Part print with two shaded views. Sizes in mm from the minimum x, y, z corner. A direction names the side the tool comes from. Coordinates: 2 decimals unless noted, no trailing zeros. Loops run counter-clockwise (first coordinate to the right, second up) from the corner with the lowest first, then second, coordinate; pieces in that order, holes last. Notation, with made-up numbers: (-35, 42) -> (-17, 42) arc R23 ccw to (-17, 76) -> close; hole circle Ø3 at (26, -13). An arc over 180 degrees is marked (long way). Return JSON: item names as keys, results as strings. Group by question number.
(1) Saw through at A-A on z = 29. Write the cut outline in (x, y).
(2) Tool access for the marked faces 5, 6 and 7: list every direction of +Z, -Z, +X, -X, +Y, -Y with a clear straight run to the whole face (end or side of a thin tool).
(3) Saw through at C-C on x = 29. Write the cut outline in (y, z).
(4) Saw through at B-B on y = 20.9. Write the cut outline in (x, z).
(5) Flat gauge pins, fed straight in: pin 1 Ø4 at (x, y) = (33.4, 32.4) entering from +Z; pin 2 Ø9 at (x, z) = (7, 11.5) entering from +Y; pin 3 Ø6.5 at (x, z) = (37.8, 29) entering from +Y. Where does each tip first touch, or does it go through?
(6) Probe L1, parallel to Z at x = 37.8, y = 1.05; L2, parallel to Z at x = 6, y = 5; L3, parallel to X at y = 20.9, z = 1.1. List the from-to ranges inside material, lowest first.
(7) Mould opens along Z. For the marked faces 1, 2, 3 and 4 say: pulls with the +Z half, pulls with the -Z half, needs draft (parallel to the pull), parting line crosses it, or undercut.
(8) Saw through at D-D on x = 4.5. Write the cut outline in (y, z).
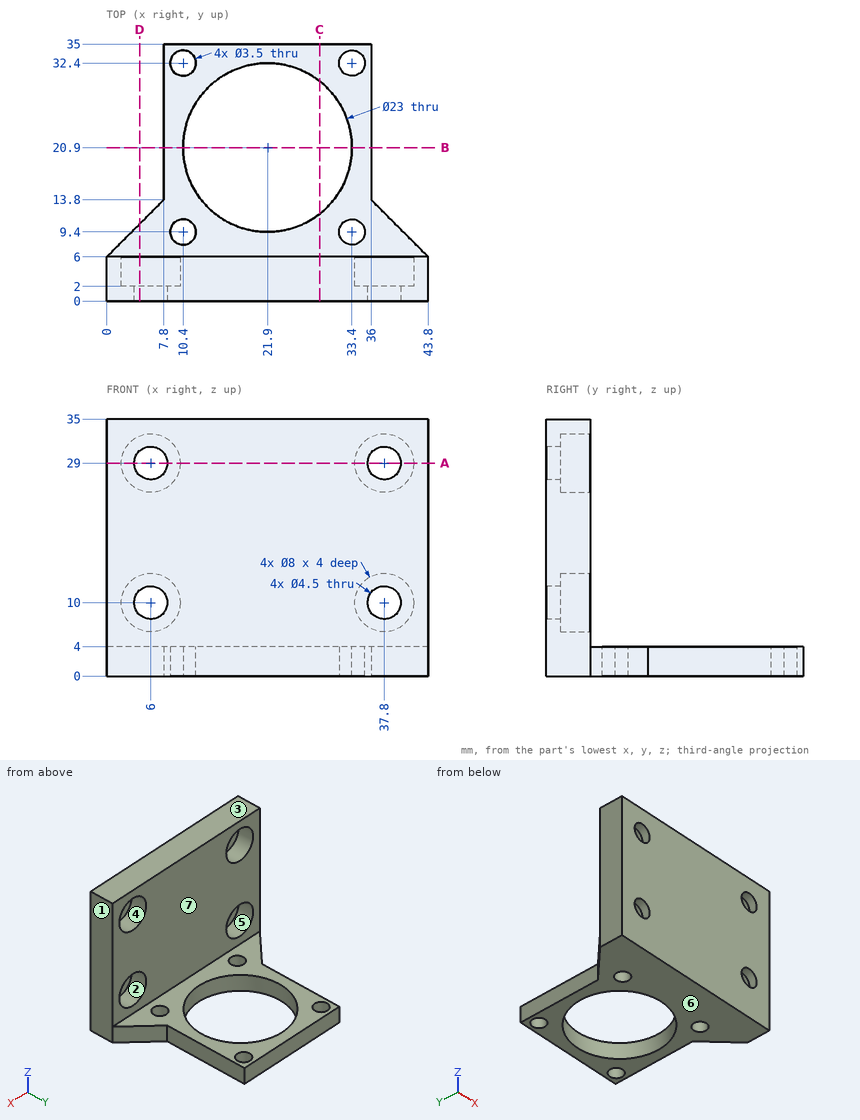
Geometry results:
{
 "1": {"outline": "(0, 0) -> (3.75, 0) -> (3.75, 2) -> (2, 2) -> (2, 6) -> (0, 6) -> close; (8.25, 0) -> (35.55, 0) -> (35.55, 2) -> (33.8, 2) -> (33.8, 6) -> (10, 6) -> (10, 2) -> (8.25, 2) -> close; (40.05, 0) -> (43.8, 0) -> (43.8, 6) -> (41.8, 6) -> (41.8, 2) -> (40.05, 2) -> close"},
 "2": {"face 5": "+Y", "face 6": "-Z, +X, -X, +Y, -Y", "face 7": "+Z, +X, -X, +Y"},
 "3": {"outline": "(0, 0) -> (11.85, 0) -> (11.85, 4) -> (6, 4) -> (6, 35) -> (0, 35) -> close; (29.95, 0) -> (35, 0) -> (35, 4) -> (29.95, 4) -> close"},
 "4": {"outline": "(7.8, 0) -> (10.4, 0) -> (10.4, 4) -> (7.8, 4) -> close; (33.4, 0) -> (36, 0) -> (36, 4) -> (33.4, 4) -> close"},
 "5": {"pin 1": "z = 4", "pin 2": "y = 6", "pin 3": "y = 2"},
 "6": {"L1": "0 to 7.75, 12.25 to 26.75, 31.25 to 35", "L2": "0 to 6, 14 to 25, 33 to 35", "L3": "7.8 to 10.4, 33.4 to 36"},
 "7": {"face 1": "needs draft", "face 2": "undercut", "face 3": "pulls with the +Z half", "face 4": "undercut"},
 "8": {"outline": "(0, 0) -> (10.5, 0) -> (10.5, 4) -> (6, 4) -> (6, 6.29) -> (2, 6.29) -> (2, 8.32) -> (0, 8.32) -> close; (0, 11.68) -> (2, 11.68) -> (2, 13.71) -> (6, 13.71) -> (6, 25.29) -> (2, 25.29) -> (2, 27.32) -> (0, 27.32) -> close; (0, 30.68) -> (2, 30.68) -> (2, 32.71) -> (6, 32.71) -> (6, 35) -> (0, 35) -> close"}
}
